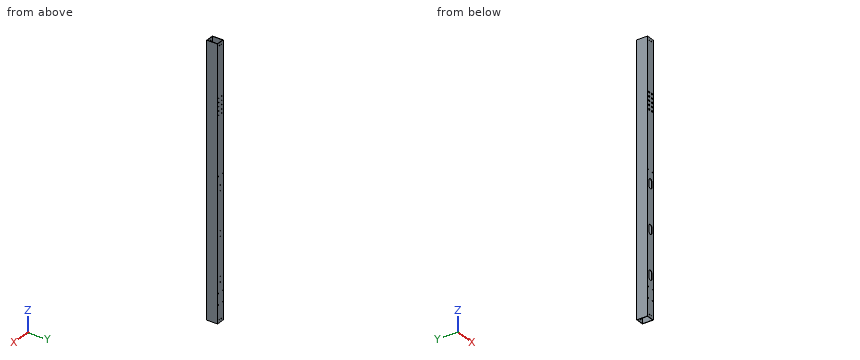
```python
from build123d import *

# Parameters (mm, degrees)
SKETCH_1_W             = 30
SKETCH_1_H             = 40
SKETCH_1_W_2           = 27
SKETCH_1_H_2           = 37
EXTRUDE_1_DEPTH        = 980
SKETCH_2_R             = 1.5
CUT_EXTRUDE_1_DEPTH    = 1040
SKETCH_3_R             = 1.5
CUT_EXTRUDE_2_DEPTH    = 981.930680527
SKETCH_4_R             = 1.5
CUT_EXTRUDE_3_DEPTH    = 981.930680527
SKETCH_5_R             = 1.5
CUT_EXTRUDE_4_DEPTH    = 981.930680527
CUT_EXTRUDE_6_DEPTH    = 10
SKETCH_9_R             = 3.25
CUT_EXTRUDE_7_DEPTH    = 10
PATTERN_LINEAR_1_COUNT = 4
PATTERN_LINEAR_1_PITCH = 15


with BuildPart() as part:
    # Sketch 1 → Extrude 1 (new body)
    with BuildSketch(Plane.XY):
        Rectangle(SKETCH_1_W, SKETCH_1_H)
        Rectangle(SKETCH_1_W_2, SKETCH_1_H_2, mode=Mode.SUBTRACT)
    extrude(amount=EXTRUDE_1_DEPTH)

    # Sketch 2 → Cut-Extrude 1 (cut)
    with BuildSketch(Plane(origin=(0, 20, 0), x_dir=(-1, 0, 0), z_dir=(0, -1, 0))):
        with Locations(Location((11, -65, 0), (0, 0, 180))):
            Circle(SKETCH_2_R)
        with Locations(Location((-11, -65, 0), (0, 0, 270))):
            Circle(SKETCH_2_R)
        with Locations(Location((11, -515, 0), (0, 0, 180))):
            Circle(SKETCH_2_R)
        with Locations(Location((-11, -515, 0), (0, 0, 270))):
            Circle(SKETCH_2_R)
        with Locations(Location((11, -105, 0), (0, 0, 180))):
            Circle(SKETCH_2_R)
        with Locations(Location((-11, -105, 0), (0, 0, 270))):
            Circle(SKETCH_2_R)
    extrude(amount=CUT_EXTRUDE_1_DEPTH, mode=Mode.SUBTRACT)

    # Sketch 3 → Cut-Extrude 2 (cut, through all)
    with BuildSketch(Plane(origin=(0, 20, 0), x_dir=(-1, 0, 0), z_dir=(0, -1, 0))):
        with Locations(Location((5, -10, 0), (0, 0, 270))):
            Circle(SKETCH_3_R)
        with Locations(Location((-5, -10, 0), (0, 0, 270))):
            Circle(SKETCH_3_R)
        with Locations(Location((-5, -970, 0), (0, 0, 270))):
            Circle(SKETCH_3_R)
        with Locations(Location((5, -970, 0), (0, 0, 270))):
            Circle(SKETCH_3_R)
    extrude(amount=CUT_EXTRUDE_2_DEPTH, mode=Mode.SUBTRACT)

    # Sketch 4 → Cut-Extrude 3 (cut, through all)
    with BuildSketch(Plane(origin=(0, 20, 0), x_dir=(-1, 0, 0), z_dir=(0, -1, 0))):
        with Locations(Location((-8.27006126, -772.5, 0), (0, 0, 270))):
            Circle(SKETCH_4_R)
        with Locations(Location((6.72993874, -772.5, 0), (0, 0, 270))):
            Circle(SKETCH_4_R)
        with Locations(Location((6.72993874, -787.5, 0), (0, 0, 270))):
            Circle(SKETCH_4_R)
        with Locations(Location((-8.27006126, -787.5, 0), (0, 0, 270))):
            Circle(SKETCH_4_R)
    cut_extrude_3 = extrude(amount=CUT_EXTRUDE_3_DEPTH, mode=Mode.SUBTRACT)

    # Sketch 5 → Cut-Extrude 4 (cut, through all)
    with BuildSketch(Plane(origin=(0, 20, 0), x_dir=(-1, 0, 0), z_dir=(0, -1, 0))):
        with Locations(Location((0, -140, 0), (0, 0, 270))):
            Circle(SKETCH_5_R)
        with Locations(Location((0, -160, 0), (0, 0, 270))):
            Circle(SKETCH_5_R)
        with Locations(Location((0, -300, 0), (0, 0, 270))):
            Circle(SKETCH_5_R)
        with Locations(Location((0, -320, 0), (0, 0, 270))):
            Circle(SKETCH_5_R)
        with Locations(Location((0, -480, 0), (0, 0, 270))):
            Circle(SKETCH_5_R)
        with Locations(Location((0, -460, 0), (0, 0, 270))):
            Circle(SKETCH_5_R)
    extrude(amount=CUT_EXTRUDE_4_DEPTH, mode=Mode.SUBTRACT)

    # Sketch 8 → Cut-Extrude 6 (cut)
    with BuildSketch(Plane.XZ.offset(20)):
        with BuildLine():
            Line((7.5, 160), (7.5, 140))
            ThreePointArc((7.5, 140), (0, 132.5), (-7.5, 140))
            Line((-7.5, 140), (-7.5, 160))
            ThreePointArc((-7.5, 160), (0, 167.5), (7.5, 160))
        make_face()
        with BuildLine():
            Line((7.5, 480), (7.5, 460))
            ThreePointArc((7.5, 460), (0, 452.5), (-7.5, 460))
            Line((-7.5, 460), (-7.5, 480))
            ThreePointArc((-7.5, 480), (0, 487.5), (7.5, 480))
        make_face()
        with BuildLine():
            Line((7.5, 320), (7.5, 300))
            ThreePointArc((7.5, 300), (0, 292.5), (-7.5, 300))
            Line((-7.5, 300), (-7.5, 320))
            ThreePointArc((-7.5, 320), (0, 327.5), (7.5, 320))
        make_face()
    extrude(amount=-CUT_EXTRUDE_6_DEPTH, mode=Mode.SUBTRACT)

    # Sketch 9 → Cut-Extrude 7 (cut)
    with BuildSketch(Plane.XZ.offset(20)):
        with Locations(Location((-6.72993874, 787.5, 0), (0, 0, 270))):
            Circle(SKETCH_9_R)
        with Locations(Location((-6.72993874, 772.5, 0), (0, 0, 270))):
            Circle(SKETCH_9_R)
        with Locations(Location((8.27006126, 772.5, 0), (0, 0, 270))):
            Circle(SKETCH_9_R)
        with Locations(Location((8.27006126, 787.5, 0), (0, 0, 270))):
            Circle(SKETCH_9_R)
    cut_extrude_7 = extrude(amount=-CUT_EXTRUDE_7_DEPTH, mode=Mode.SUBTRACT)

    # Pattern Linear 1: Cut-Extrude 3, Cut-Extrude 7 ×4
    with Locations(*[(0, 0, -i * PATTERN_LINEAR_1_PITCH) for i in range(1, PATTERN_LINEAR_1_COUNT)]):
        add(cut_extrude_3, mode=Mode.SUBTRACT)
        add(cut_extrude_7, mode=Mode.SUBTRACT)


solid = part.part
```
Geometry check sheet. Reference: the model listing, model coordinates, mm. Round coordinates to 2 decimals unless told otherwise and drop trailing zeros. Order: outer loops, then holes, each group sorted by start corner. A loop starts at its lowest first (then second) coordinate and runs counter-clockwise, first axis right, second up. Notation, with made-up numbers: M -33.75,43 L 19.25,43 A36 cw 19.25,79 Z; hole C 51.5,56 d10. An arc over 180 degrees is marked long. Answer as CSV lines item,"result".
1) Sectioned sample at A-A on y = -2.5. Record the cut outline in (x, z), and give its area (3 significant figures).
Entries:
outline,"M -15,0 L -13.5,0 L -13.5,980 L -15,980 Z; M 13.5,0 L 15,0 L 15,980 L 13.5,980 Z"
area,"2,940 mm2"
2) Sectioned sample at B-B on z = 410. Record the cut outline in (x, y), and give its area (3 significant figures).
Entries:
outline,"M -15,-20 L 15,-20 L 15,20 L -15,20 Z; hole M -13.5,-18.5 L 13.5,-18.5 L 13.5,18.5 L -13.5,18.5 Z"
area,"201 mm2"
3) Gauge pin test, flat end, axial feed: pin 1 Ø4 at (x, z) = (8.27, 757.5) entering from -Y. Record the tip position at first contact, or that the pin passes through.
Entries:
pin 1,"y = 18.5"
4) Thickness scan on probe 1 along Z at (x, y) = (11, 19.5); probe 2 along X at (y, z) = (18.95, 772.5); probe 3 along X at (y, z) = (-19.6, 787.5). Record the ranges inside material, lowest first. Write a range as [from, to].
Entries:
probe 1,"[0, 63.5], [66.5, 103.5], [106.5, 513.5], [516.5, 980]"
probe 2,"[-15, -8.23], [-5.23, 6.77], [9.77, 15]"
probe 3,"[-15, -9.98], [-3.48, 5.02], [11.52, 15]"
